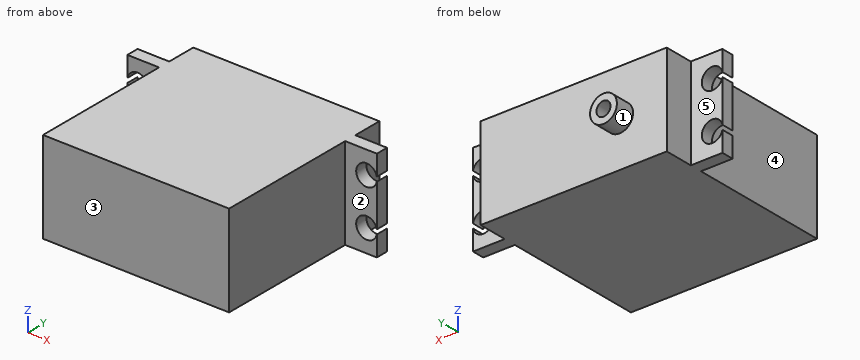
```python
from build123d import *

# Parameters (mm, degrees)
SKETCH1_W           = 40.2844
SKETCH1_H           = 19.7612
BOSS_EXTRUDE1_DEPTH = 39.4208
SKETCH2_W           = 19.7612
SKETCH2_H           = 2.667
BOSS_EXTRUDE2_DEPTH = 6.858
SKETCH3_R           = 2.2606
CUT_EXTRUDE2_DEPTH  = 44.859747411
SKETCH4_R           = 2.9083
BOSS_EXTRUDE3_DEPTH = 4.2418
SKETCH5_R           = 1.524
CUT_EXTRUDE3_DEPTH  = 7.4422


with BuildPart() as part:
    # Sketch1 → Boss-Extrude1 (new body)
    with BuildSketch(Plane(origin=(0, 0, 0), x_dir=(1, 0, 0), z_dir=(0, 1, 0))):
        Rectangle(SKETCH1_W, SKETCH1_H)
    extrude(amount=BOSS_EXTRUDE1_DEPTH)

    # Sketch2 → Boss-Extrude2 (add)
    with BuildSketch(Plane(origin=(20.1422, 0, 0), x_dir=(0, 0, -1), z_dir=(1, 0, 0))):
        with Locations((0, 31.7881)):
            Rectangle(SKETCH2_W, SKETCH2_H)
    boss_extrude2 = extrude(amount=BOSS_EXTRUDE2_DEPTH)

    # Sketch3 → Cut-Extrude2 (cut, through all)
    with BuildSketch(Plane(origin=(0, 33.1216, 0), x_dir=(1, 0, 0), z_dir=(0, 1, 0))):
        with Locations((24.7904, 5.0165)):
            Circle(SKETCH3_R)
        with Locations((24.7904, -5.0165)):
            Circle(SKETCH3_R)
    cut_extrude2 = extrude(amount=-CUT_EXTRUDE2_DEPTH, mode=Mode.SUBTRACT)

    # Mirror1: Boss-Extrude2, Cut-Extrude2 across plane
    add(boss_extrude2.mirror(Plane(origin=(0, 0, 0), x_dir=(0, 0, 1), z_dir=(1, 0, 0))))
    add(cut_extrude2.mirror(Plane(origin=(0, 0, 0), x_dir=(0, 0, 1), z_dir=(1, 0, 0))), mode=Mode.SUBTRACT)

    # Sketch4 → Boss-Extrude3 (add)
    with BuildSketch(Plane(origin=(0, 39.4208, 0), x_dir=(1, 0, 0), z_dir=(0, 1, 0))):
        with Locations(Location((-9.9441, 0, 0), (0, 0, 90))):
            Circle(SKETCH4_R)
    extrude(amount=BOSS_EXTRUDE3_DEPTH)

    # Sketch5 → Cut-Extrude3 (cut)
    with BuildSketch(Plane(origin=(0, 43.6626, 0), x_dir=(1, 0, 0), z_dir=(0, 1, 0))):
        with Locations(Location((-9.9441, 0, 0), (0, 0, 270))):
            Circle(SKETCH5_R)
    extrude(amount=-CUT_EXTRUDE3_DEPTH, mode=Mode.SUBTRACT)


solid = part.part
```
Geometry check sheet. Reference: the model listing, model coordinates, mm. Face numbers are marked on the shaded views. A direction names the side the tool comes from. Round coordinates to 2 decimals unless told otherwise and drop trailing zeros. Order: outer loops, then holes, each group sorted by start corner. A loop starts at its lowest first (then second) coordinate and runs counter-clockwise, first axis right, second up. Notation, with made-up numbers: M 36.25,-20.75 L 86.25,-20.75 A29 cw 86.25,8.25 Z; hole C 76.5,3 d11. An arc over 180 degrees is marked long. Write item = value, one per line.
Q1. Section check C-C (y = 29). Enter the section's corners in (x, z).
Answer block:
outline = M -20.14,-9.88 L 20.14,-9.88 L 20.14,9.88 L -20.14,9.88 Z
Q2. Section check D-D (x = -19). Enter the section's corners in (y, z), plus the area to 3 significant figures.
Answer block:
outline = M 0,-9.88 L 39.42,-9.88 L 39.42,9.88 L 0,9.88 Z
area = 779 mm^2
Q3. Section check A-A (z = 0). Enter the section's corners in (x, y), plus the area to 3 significant figures.
Answer block:
outline = M -27,30.45 L -20.14,30.45 L -20.14,0 L 20.14,0 L 20.14,30.45 L 27,30.45 L 27,33.12 L 20.14,33.12 L 20.14,39.42 L -7.04,39.42 L -7.04,43.66 L -8.42,43.66 L -8.42,36.22 L -11.47,36.22 L -11.47,43.66 L -12.85,43.66 L -12.85,39.42 L -20.14,39.42 L -20.14,33.12 L -27,33.12 Z
area = 1,630 mm^2
Q4. Section check B-B (z = 3.75). Enter the section's corners in (x, y).
Answer block:
outline = M -27,30.45 L -26.66,30.45 L -26.66,33.12 L -27,33.12 Z; M -22.92,30.45 L -20.14,30.45 L -20.14,0 L 20.14,0 L 20.14,30.45 L 22.92,30.45 L 22.92,33.12 L 20.14,33.12 L 20.14,39.42 L -20.14,39.42 L -20.14,33.12 L -22.92,33.12 Z; M 26.66,30.45 L 27,30.45 L 27,33.12 L 26.66,33.12 Z
Q5. Scan lines: line 1 (Y direction, x = -9, z = -8.25); line 2 (X direction, y = 41.25, z = 0); line 3 (X direction, y = 11, z = 6.25). Record each from-to range of solid material in increasing order.
Answer block:
line_1 = 0 to 39.42
line_2 = -12.85 to -11.47, -8.42 to -7.04
line_3 = -20.14 to 20.14
Q6. Set-up check for the marked faces 1, 2, 3, 4 and 5: record each of +Z, -Z, +X, -X, +Y, -Y from which the full face is reachable in a straight line by a thin tool's end or side.
Answer block:
face_1 = +Y
face_2 = +Z, -Z, +X, -Y
face_3 = +Z, -Z, +X, -X, -Y
face_4 = +Z, -Z, -X, -Y
face_5 = +Z, -Z, -X, +Y
Q7. Depth check by flat-ended pin: pin 1 Ø3.5 at (x, z) = (-9.94, 0) entering from +Y; pin 2 Ø6 at (y, z) = (18.5, -4.5) entering from -X; pin 3 Ø5 at (x, z) = (-17.5, -1) entering from +Y; pin 4 Ø5.5 at (x, z) = (23.5, 4) entering from -Y. Enter the tip coordinate at first touch or a pass-through.
Answer block:
pin_1 = 43.66
pin_2 = -20.14
pin_3 = 39.42
pin_4 = 30.45
